Build history of the part. All positions in model axes, mm. Face numbers are marked on the shaded views. A direction names the side the tool comes from. Round coordinates to 2 decimals unless told otherwise and drop trailing zeros. Loops run counter-clockwise (first coordinate to the right, second up) from the corner with the lowest first, then second, coordinate; pieces in that order, holes last. Notation, with made-up numbers: (-28, 10.25) - (-18, 10.25) arc R10 cw to (-18, 25.25) - close; hole circle Ø5 at (-5.5, -28). An arc over 180 degrees is marked (long way). Put each result on its own line as item: value. Start each with the question number.
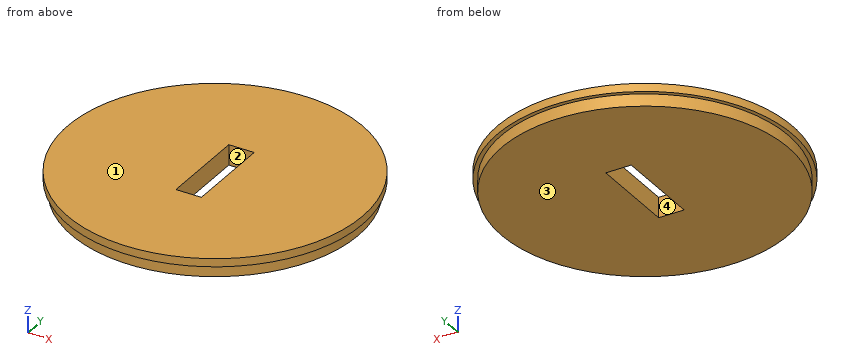
from build123d import *

# Parameters (mm, degrees)
F0_R     = 35.3
F1_DEPTH = 3
F3_R     = 36.3
F4_DEPTH = 2
F5_W     = 6.26
F5_H     = 21.66028
F6_DEPTH = 25


with BuildPart() as f1:
    # F0 (on Top) → F1 (new body)
    with BuildSketch(Plane.XY):
        Circle(F0_R)
    extrude(amount=F1_DEPTH)

    # F3 (on offset) → F4 (join)
    with BuildSketch(Plane.XY.offset(3)):
        Circle(F3_R)
    extrude(amount=F4_DEPTH)

    # F5 (on face) → F6 (cut)
    with BuildSketch(Plane.XY.offset(5)):
        with Locations((0, -0.00014)):
            Rectangle(F5_W, F5_H)
    extrude(amount=-F6_DEPTH, mode=Mode.SUBTRACT)


solid = f1.part
Item 1: Which spindle directions (+Z, -Z, +X, -X, +Y, -Y) get a long thin tool onto all of the face, cutting with end or side? Do the marked faces 3 and 4. Say none if no direction does.
Item 2: Slice it at A-A (x = 0). Give the cut face in (y, z).
Item 3: Two-plate mould, pull along X, no slides. Class the marked faces 1 and 2: pulls with the +X half, pulls with the -X half, needs draft (parallel to the pull), parting line crosses it, or undercut.
Item 4: Slice it at C-C (z = 1.95). Give the cut face in (x, y), plus the area to 3 significant figures.
Item 5: Drop flat-ended pins along their axis: pin 1 Ø5 at (x, y) = (-13.5, 3) entering from -Z; pin 2 Ø2.5 at (x, z) = (1, 3.5) entering from +Y; pin 3 Ø2 at (x, z) = (13, 3.5) entering from +Y; pin 4 Ø2.5 at (y, z) = (-1.5, 1.5) entering from -X. Give the stop position or say it passes through.
Item 6: Slice it at D-D (y = -29). Give the cut face in (x, z).
Item 7: Drill centre lines: probe 1 along Y at (x, z) = (0, 4.55); probe 2 along Y at (x, z) = (-1, 0.65); probe 3 along X at (y, z) = (10, 3.5). Where is each one in solid material? Low to high. Write a range as [from, to].
Item 8: Slice it at B-B (y = 0). Give the cut face in (x, z).
Computed values:
1. face 3: -Z, +X, -X, +Y, -Y
1. face 4: +Z, -Z
2. outline: (-36.3, 3) - (-35.3, 3) - (-35.3, 0) - (-10.83, 0) - (-10.83, 5) - (-36.3, 5) - close; (10.83, 0) - (35.3, 0) - (35.3, 3) - (36.3, 3) - (36.3, 5) - (10.83, 5) - close
3. face 1: needs draft
3. face 2: undercut
4. outline: circle Ø70.6 at (0, 0); hole (-3.13, -10.83) - (3.13, -10.83) - (3.13, 10.83) - (-3.13, 10.83) - close
4. area: 3,780 mm^2
5. pin 1: stops at z = 0
5. pin 2: stops at y = 36.3
5. pin 3: stops at y = 34.26
5. pin 4: stops at x = -35.3
6. outline: (-21.83, 3) - (-20.13, 3) - (-20.13, 0) - (20.13, 0) - (20.13, 3) - (21.83, 3) - (21.83, 5) - (-21.83, 5) - close
7. probe 1: y = [-36.3, -10.83], [10.83, 36.3]
7. probe 2: y = [-35.29, -10.83], [10.83, 35.29]
7. probe 3: x = [-34.9, -3.13], [3.13, 34.9]
8. outline: (-36.3, 3) - (-35.3, 3) - (-35.3, 0) - (-3.13, 0) - (-3.13, 5) - (-36.3, 5) - close; (3.13, 0) - (35.3, 0) - (35.3, 3) - (36.3, 3) - (36.3, 5) - (3.13, 5) - close
